Verification items for the finished model (mm, model axes). Coordinates: 2 decimals unless noted, no trailing zeros. Write each loop counter-clockwise with the first axis right and the second up, starting at its lowest first coordinate (ties: lowest second). Pieces come first, ordered by that corner, then holes. Notation, with made-up numbers: (-38, 82.5) -> (-13, 82.5) arc R20 ccw to (-13, 93.5) -> close; hole circle Ø7 at (20, 27.25). An arc over 180 degrees is marked (long way). Write item = value, one per line. Start each with the question number.
(1) Section check B-B (z = 10). Record the cut outline in (x, y), plus the area to 3 significant figures.
(2) Section check A-A (x = -10). Record the cut outline in (y, z), plus the area to 3 significant figures.
(3) Section check C-C (y = -0.2). Record the cut outline in (x, z), plus the area to 3 significant figures.
(4) Material ranges on probe 1 along X at (y, z) = (-0.1, -11); probe 2 along Z at (x, y) = (-10, 0); probe 3 along Z at (x, y) = (10.75, -0.3), recorded low to high. Write a range as [from, to].
(5) Gauge pin test, flat end, axial feed: pin 1 Ø5 at (x, z) = (-10, -11) entering from -Y. Record the tip position at first contact, or that the pin passes through.
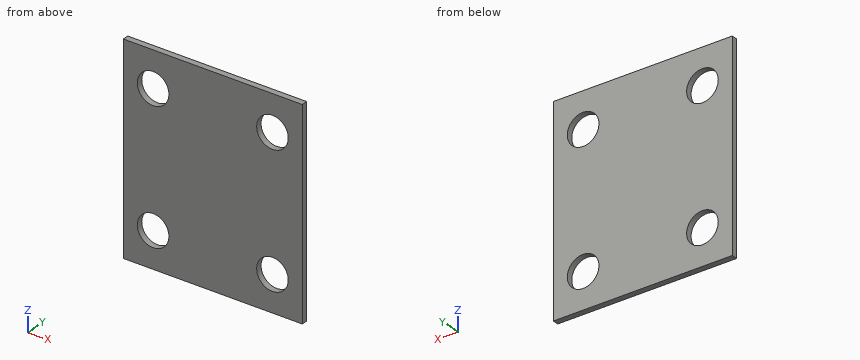
```python
from build123d import *

# Parameters (mm, degrees)
BASE_FLANGE1_START     = -0.5
BASE_FLANGE1_OUTLINE_W = 30
BASE_FLANGE1_OUTLINE_H = 34
BASE_FLANGE1_DEPTH     = 1
M5_CLEARANCE_HOLE2_D   = 5.3


# Read off the part's stored shape, not the designer's step: Base-Flange1
with BuildPart() as part:
    # Base-Flange1 outline → Base-Flange1 (new body)
    with BuildSketch(Plane(origin=(0, 0, 0), x_dir=(1, 0, 0), z_dir=(0, 1, 0)).offset(BASE_FLANGE1_START)):
        Rectangle(BASE_FLANGE1_OUTLINE_W, BASE_FLANGE1_OUTLINE_H)
    extrude(amount=BASE_FLANGE1_DEPTH)

    # M5 Clearance Hole2 (through all)
    with Locations(Plane(origin=(0, 0.5, 0), x_dir=(1, 0, 0), z_dir=(0, 1, 0))):
        with Locations((-10, -11), (10, -11), (-10, 11), (10, 11)):
            Hole(M5_CLEARANCE_HOLE2_D / 2)


solid = part.part
```
Response:
q1.outline = (-15, -0.5) -> (-12.45, -0.5) -> (-12.45, 0.5) -> (-15, 0.5) -> close; (-7.55, -0.5) -> (7.55, -0.5) -> (7.55, 0.5) -> (-7.55, 0.5) -> close; (12.45, -0.5) -> (15, -0.5) -> (15, 0.5) -> (12.45, 0.5) -> close
q1.area = 20.2 mm2
q2.outline = (-0.5, -17) -> (0.5, -17) -> (0.5, -13.65) -> (-0.5, -13.65) -> close; (-0.5, -8.35) -> (0.5, -8.35) -> (0.5, 8.35) -> (-0.5, 8.35) -> close; (-0.5, 13.65) -> (0.5, 13.65) -> (0.5, 17) -> (-0.5, 17) -> close
q2.area = 23.4 mm2
q3.outline = (-15, -17) -> (15, -17) -> (15, 17) -> (-15, 17) -> close; hole circle Ø5.3 at (-10, -11); hole circle Ø5.3 at (-10, 11); hole circle Ø5.3 at (10, -11); hole circle Ø5.3 at (10, 11)
q3.area = 932 mm2
q4.probe_1 = [-15, -12.65], [-7.35, 7.35], [12.65, 15]
q4.probe_2 = [-17, -13.65], [-8.35, 8.35], [13.65, 17]
q4.probe_3 = [-17, -13.54], [-8.46, 8.46], [13.54, 17]
q5.pin_1 = through
